Check sheet for the modelled part. Datum: model origin and axes. Units: mm. A direction names the side the tool comes from. Round coordinates to 2 decimals unless told otherwise and drop trailing zeros. Loops run counter-clockwise (first coordinate to the right, second up) from the corner with the lowest first, then second, coordinate; pieces in that order, holes last. Notation, with made-up numbers: M 25,3.5 L 61,3.5 A28 cw 61,32.5 Z; hole C 57,53 d10. An arc over 180 degrees is marked long. Write item = value, one per line. Start each with the question number.
(1) Cross-section at B-B on x = 23.5. Record the boundary of the cut face in (y, z).
(2) Mould release check, pull along X, two halves, no side actions. Record for faces 3 (the face through (23, 1, -9)), 4 (the face through (29.07, 0.06, -6.08)), 5 (the face through (-19.5, 1, -12)), 6 (the face through (-29.12, 1.48, -6.06)): pulls with the +X half, pulls with the -X half, needs draft (parallel to the pull), parting line crosses it, or undercut.
(3) Cross-section at A-A on y = 0.8. Record the boundary of the cut face in (x, z), plus the area to 3 significant figures.
(4) Set-up check for faces 1 (the face through (25.5, 1, -12)), 2 (the face through (0, 0, -8)): record each of +Z, -Z, +X, -X, +Y, -Y from which the full face is reachable in a straight line by a thin tool's end or side.
(5) Scan lines: L1, parallel to X at y = 0.25, z = -11; L2, parallel to X at y = 2.35, z = -14; L3, parallel to Z at x = -21.5, y = 2.6. Record each from-to range of solid material in increasing order. Write a range as from..to.
(6) Go/stop test with flat-tipped pins: P1, Ø0.8, axis at x = -22, y = 1.5, coming from the -Z side; P2, Ø1, axis at y = 1.5, z = -3.5, coming from the +X side; P3, Ø0.8, axis at y = 2, z = -13.5, coming from the +X side. Record where each tip stops, or that it passes through.
from build123d import *

# Parameters (mm, degrees)
BOSS_EXTRUDE1_DEPTH = 3
FILLET1_R           = 0.2


with BuildPart() as part:
    # Sketch1 → Boss-Extrude1 (new body)
    with BuildSketch(Plane(origin=(0, 0, 0), x_dir=(1, 0, 0), z_dir=(0, 1, 0))):
        with BuildLine():
            Line((19.5, 15), (-19.5, 15))
            Line((-19.5, 15), (-19.5, 10))
            ThreePointArc((-19.5, 10), (-19.792893219, 9.292893219), (-20.5, 9))
            Line((-20.5, 9), (-24.5, 9))
            ThreePointArc((-24.5, 9), (-25.207106781, 9.292893219), (-25.5, 10))
            Line((-25.5, 10), (-25.5, 15))
            Line((-25.5, 15), (-28.5, 15))
            ThreePointArc((-28.5, 15), (-29.914213562, 14.414213562), (-30.5, 13))
            Line((-30.5, 13), (-30.5, 10))
            Line((-30.5, 10), (-27.703132054, 2.008948726))
            ThreePointArc((-27.703132054, 2.008948726), (-26.60747838, 0.553251768), (-24.871556985, 0))
            Line((-24.871556985, 0), (24.871556985, 0))
            ThreePointArc((24.871556985, 0), (26.60747838, 0.553251768), (27.703132054, 2.008948726))
            Line((27.703132054, 2.008948726), (30.5, 10))
            Line((30.5, 10), (30.5, 13))
            ThreePointArc((30.5, 13), (29.914213562, 14.414213562), (28.5, 15))
            Line((28.5, 15), (25.5, 15))
            Line((25.5, 15), (25.5, 10))
            ThreePointArc((25.5, 10), (25.207106781, 9.292893219), (24.5, 9))
            Line((24.5, 9), (20.5, 9))
            ThreePointArc((20.5, 9), (19.792893219, 9.292893219), (19.5, 10))
            Line((19.5, 10), (19.5, 15))
        make_face()
    extrude(amount=BOSS_EXTRUDE1_DEPTH)

    # Fillet1
    fillet1_edges = [part.edges().sort_by_distance(p)[0] for p in [
        (-25.207106781, 3, -9.292893219),
        (-25.5, 3, -12.5),
        (-27, 3, -15),
        (-19.5, 0, -12.5),
        (-29.914213562, 3, -14.414213562),
        (0, 0, -15),
        (19.5, 0, -12.5),
        (19.792893219, 0, -9.292893219),
        (22.5, 0, -9),
        (25.207106781, 0, -9.292893219),
        (25.5, 0, -12.5),
        (27, 0, -15),
        (-30.5, 3, -11.5),
        (29.914213562, 0, -14.414213562),
        (30.5, 0, -11.5),
        (29.101566027, 0, -6.004474363),
        (26.60747838, 0, -0.553251768),
        (0, 0, 0),
        (-26.60747838, 0, -0.553251768),
        (-29.101566027, 0, -6.004474363),
        (-30.5, 0, -11.5),
        (-29.101566027, 3, -6.004474363),
        (-29.914213562, 0, -14.414213562),
        (-27, 0, -15),
        (-25.5, 0, -12.5),
        (-25.207106781, 0, -9.292893219),
        (-22.5, 0, -9),
        (-19.792893219, 0, -9.292893219),
        (-26.60747838, 3, -0.553251768),
        (0, 3, 0),
        (26.60747838, 3, -0.553251768),
        (-19.5, 1.5, -15),
        (19.5, 1.5, -15),
        (25.5, 1.5, -15),
        (-25.5, 1.5, -15),
        (29.101566027, 3, -6.004474363),
        (-19.792893219, 3, -9.292893219),
        (30.5, 3, -11.5),
        (29.914213562, 3, -14.414213562),
        (27, 3, -15),
        (25.5, 3, -12.5),
        (25.207106781, 3, -9.292893219),
        (22.5, 3, -9),
        (19.792893219, 3, -9.292893219),
        (19.5, 3, -12.5),
        (0, 3, -15),
        (-19.5, 3, -12.5),
        (-22.5, 3, -9),
    ]]
    fillet(fillet1_edges, radius=FILLET1_R)


solid = part.part
Result:
q1.outline = M 0,-8.8 A0.2 ccw 0.2,-9 L 2.8,-9 A0.2 ccw 3,-8.8 L 3,-0.2 A0.2 ccw 2.8,0 L 0.2,0 A0.2 ccw 0,-0.2 Z
q2.face_3 = undercut
q2.face_4 = pulls with the +X half
q2.face_5 = undercut
q2.face_6 = pulls with the -X half
q3.outline = M -30.5,-13 A2 ccw -28.5,-15 L -25.7,-15 A0.2 ccw -25.5,-14.8 L -25.5,-10 A1 cw -24.5,-9 L -20.5,-9 A1 cw -19.5,-10 L -19.5,-14.8 A0.2 ccw -19.3,-15 L 19.3,-15 A0.2 ccw 19.5,-14.8 L 19.5,-10 A1 cw 20.5,-9 L 24.5,-9 A1 cw 25.5,-10 L 25.5,-14.8 A0.2 ccw 25.7,-15 L 28.5,-15 A2 ccw 30.5,-13 L 30.5,-10 L 27.7,-2.01 A3 ccw 24.87,0 L -24.87,0 A3 ccw -27.7,-2.01 L -30.5,-10 Z
q3.area = 805 mm^2
q4.face_1 = -Z, +Y, -Y
q4.face_2 = +Z, -Z, +X, -X, -Y
q5.L1 = -30.5..-25.5, -19.5..19.5, 25.5..30.5
q5.L2 = -30.23..-25.5, -19.5..19.5, 25.5..30.23
q5.L3 = -9..0
q6.P1 = -9
q6.P2 = 28.4
q6.P3 = 30.5
